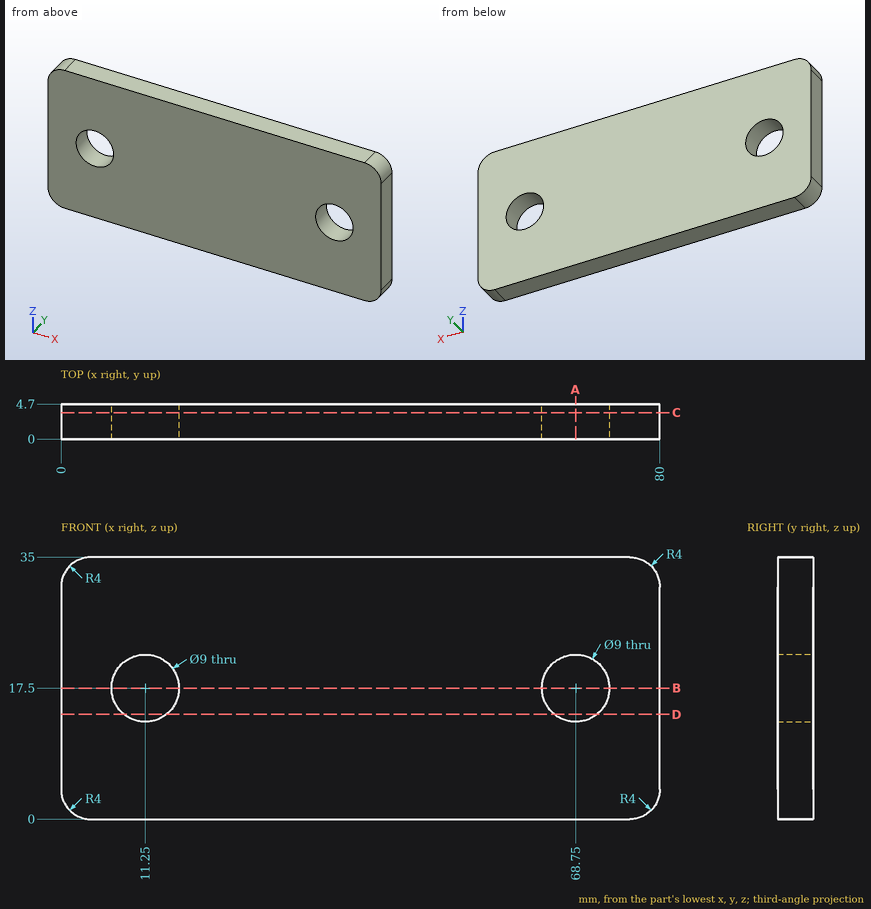
Geometry: see drawing. Coordinates: mm, zero at the bounding-box minimum. Give positions to 0.01 mm unless a question says otherwise; leave off trailing zeros. Loops run counter-clockwise (first coordinate to the right, second up) from the corner with the lowest first, then second, coordinate; pieces in that order, holes last. Notation, with made-up numbers: (73.5, -23) -> (100.5, -23) arc R36 ccw to (100.5, 13) -> close; hole circle Ø9 at (34.25, 41). An arc over 180 degrees is marked (long way). Use CSV: the item, a comma, the result in double quotes.
(1) Ray query, line 1 along X through (y, z) = (3.2, 17.5); line 2 along Z through (x, y) = (68.75, 2.65); line 3 along X through (y, z) = (3.25, 20.5). Return the intervals inside material, ascending. Write a range as [from, to].
From the geometry:
line 1,"[0, 6.75], [15.75, 64.25], [73.25, 80]"
line 2,"[0, 13], [22, 35]"
line 3,"[0, 7.9], [14.6, 65.4], [72.1, 80]"
(2) Cut plane B-B (z = 17.5). Output: boundary loops of the cut face in (x, y), plus the area to 3 significant figures.
From the geometry:
outline,"(0, 0) -> (6.75, 0) -> (6.75, 4.7) -> (0, 4.7) -> close; (15.75, 0) -> (64.25, 0) -> (64.25, 4.7) -> (15.75, 4.7) -> close; (73.25, 0) -> (80, 0) -> (80, 4.7) -> (73.25, 4.7) -> close"
area,"291 mm^2"
(3) Cut plane D-D (z = 14). Output: boundary loops of the cut face in (x, y).
From the geometry:
outline,"(0, 0) -> (8.42, 0) -> (8.42, 4.7) -> (0, 4.7) -> close; (14.08, 0) -> (65.92, 0) -> (65.92, 4.7) -> (14.08, 4.7) -> close; (71.58, 0) -> (80, 0) -> (80, 4.7) -> (71.58, 4.7) -> close"
(4) First-contact query: P1, Ø1, axis at x = 18.5, z = 24.5, coming from the -Y side. Flat tip, straight axial feed; report the tip coordinate or a pass-through.
From the geometry:
P1,"y = 0"
(5) Cut plane C-C (y = 3.55). Output: boundary loops of the cut face in (x, z).
From the geometry:
outline,"(0, 4) arc R4 ccw to (4, 0) -> (76, 0) arc R4 ccw to (80, 4) -> (80, 31) arc R4 ccw to (76, 35) -> (4, 35) arc R4 ccw to (0, 31) -> close; hole circle Ø9 at (11.25, 17.5); hole circle Ø9 at (68.75, 17.5)"
(6) Cut plane A-A (x = 68.75). Output: boundary loops of the cut face in (y, z), plus the area to 3 significant figures.
From the geometry:
outline,"(0, 0) -> (4.7, 0) -> (4.7, 13) -> (0, 13) -> close; (0, 22) -> (4.7, 22) -> (4.7, 35) -> (0, 35) -> close"
area,"122 mm^2"
